Source: CAD feature listing. Evaluate the final solid. Frame: model axes, mm. A direction names the side the tool comes from. Coordinates: 2 decimals unless noted, no trailing zeros. Loops run counter-clockwise (first coordinate to the right, second up) from the corner with the lowest first, then second, coordinate; pieces in that order, holes last.
```python
from build123d import *

# Parameters (mm, degrees)
ESQUISSE1_W        = 5
ESQUISSE1_H        = 5
ESQUISSE1_W_2      = 7.5
ESQUISSE1_R        = 1.5
ESQUISSE1_R_2      = 0.875
ESQUISSE1_R_3      = 3.5
BOSS_EXTRU_1_DEPTH = 5


with BuildPart() as part:
    # Esquisse1 → Boss.-Extru.1 (new body)
    # profile 1 of 4: a face of its own
    with BuildSketch(Plane.XY):
        with BuildLine():
            Line((-8, 5), (-8, -10))
            Line((-8, -10), (18, -10))
            Line((18, -10), (18, 0))
            Line((18, 0), (25, 0))
            Line((25, 0), (30, 19))
            Line((30, 19), (45, 19))
            Line((45, 19), (45, 34))
            Line((45, 34), (60, 34))
            ThreePointArc((60, 34), (67.778174593, 52.778174593), (49, 45))
            Line((49, 45), (49, 40))
            Line((49, 40), (20, 40))
            Line((20, 40), (20, 45))
            Line((20, 45), (10, 45))
            Line((10, 45), (10, 40))
            Line((10, 40), (5, 40))
            Line((5, 40), (5, 45))
            Line((5, 45), (-5, 45))
            Line((-5, 45), (-5, 40))
            Line((-5, 40), (-15, 40))
            Line((-15, 40), (-15, 21))
            Line((-15, 21), (-6, 21))
            Line((-6, 21), (-6, 24))
            Line((-6, 24), (9, 24))
            Line((9, 24), (9, 21))
            Line((9, 21), (17, 21))
            Line((17, 21), (17, 13))
            Line((17, 13), (13, 13))
            Line((13, 13), (13, 7))
            Line((13, 7), (9, 7))
            Line((9, 7), (9, 4))
            Line((9, 4), (0, 4))
            Line((0, 4), (0, 5))
            Line((0, 5), (-8, 5))
        make_face()
        with Locations((-2.5, -2.5)):
            Rectangle(ESQUISSE1_W, ESQUISSE1_H, mode=Mode.SUBTRACT)
        with Locations((9.25, -2.5)):
            Rectangle(ESQUISSE1_W_2, ESQUISSE1_H, mode=Mode.SUBTRACT)
        with Locations((35, 25)):
            Circle(ESQUISSE1_R, mode=Mode.SUBTRACT)
        with Locations((56.75, 37.35)):
            Circle(ESQUISSE1_R_2, mode=Mode.SUBTRACT)
        with Locations((60, 45)):
            Circle(ESQUISSE1_R_3, mode=Mode.SUBTRACT)
        with Locations((67.65, 41.75)):
            Circle(ESQUISSE1_R_2, mode=Mode.SUBTRACT)
        with Locations((52.35, 48.25)):
            Circle(ESQUISSE1_R_2, mode=Mode.SUBTRACT)
        with Locations((63.25, 52.65)):
            Circle(ESQUISSE1_R_2, mode=Mode.SUBTRACT)
    # profile 2 of 4: a face of its own
    with BuildSketch(Plane.XY):
        with BuildLine():
            Line((-8, 5), (-8, -10))
            Line((-8, -10), (18, -10))
            Line((18, -10), (18, 0))
            Line((18, 0), (25, 0))
            Line((25, 0), (30, 19))
            Line((30, 19), (45, 19))
            Line((45, 19), (45, 34))
            Line((45, 34), (60, 34))
            ThreePointArc((60, 34), (67.778174593, 52.778174593), (49, 45))
            Line((49, 45), (49, 40))
            Line((49, 40), (20, 40))
            Line((20, 40), (20, 45))
            Line((20, 45), (10, 45))
            Line((10, 45), (10, 40))
            Line((10, 40), (5, 40))
            Line((5, 40), (5, 45))
            Line((5, 45), (-5, 45))
            Line((-5, 45), (-5, 40))
            Line((-5, 40), (-15, 40))
            Line((-15, 40), (-15, 21))
            Line((-15, 21), (-6, 21))
            Line((-6, 21), (-6, 24))
            Line((-6, 24), (9, 24))
            Line((9, 24), (9, 21))
            Line((9, 21), (17, 21))
            Line((17, 21), (17, 13))
            Line((17, 13), (13, 13))
            Line((13, 13), (13, 7))
            Line((13, 7), (9, 7))
            Line((9, 7), (9, 4))
            Line((9, 4), (0, 4))
            Line((0, 4), (0, 5))
            Line((0, 5), (-8, 5))
        make_face()
        with Locations((-2.5, -2.5)):
            Rectangle(ESQUISSE1_W, ESQUISSE1_H, mode=Mode.SUBTRACT)
        with Locations((9.25, -2.5)):
            Rectangle(ESQUISSE1_W_2, ESQUISSE1_H, mode=Mode.SUBTRACT)
        with Locations((35, 25)):
            Circle(ESQUISSE1_R, mode=Mode.SUBTRACT)
        with Locations((56.75, 37.35)):
            Circle(ESQUISSE1_R_2, mode=Mode.SUBTRACT)
        with Locations((60, 45)):
            Circle(ESQUISSE1_R_3, mode=Mode.SUBTRACT)
        with Locations((67.65, 41.75)):
            Circle(ESQUISSE1_R_2, mode=Mode.SUBTRACT)
        with Locations((52.35, 48.25)):
            Circle(ESQUISSE1_R_2, mode=Mode.SUBTRACT)
        with Locations((63.25, 52.65)):
            Circle(ESQUISSE1_R_2, mode=Mode.SUBTRACT)
    # profile 3 of 4: a face of its own
    with BuildSketch(Plane.XY):
        with BuildLine():
            Line((-8, 5), (-8, -10))
            Line((-8, -10), (18, -10))
            Line((18, -10), (18, 0))
            Line((18, 0), (25, 0))
            Line((25, 0), (30, 19))
            Line((30, 19), (45, 19))
            Line((45, 19), (45, 34))
            Line((45, 34), (60, 34))
            ThreePointArc((60, 34), (67.778174593, 52.778174593), (49, 45))
            Line((49, 45), (49, 40))
            Line((49, 40), (20, 40))
            Line((20, 40), (20, 45))
            Line((20, 45), (10, 45))
            Line((10, 45), (10, 40))
            Line((10, 40), (5, 40))
            Line((5, 40), (5, 45))
            Line((5, 45), (-5, 45))
            Line((-5, 45), (-5, 40))
            Line((-5, 40), (-15, 40))
            Line((-15, 40), (-15, 21))
            Line((-15, 21), (-6, 21))
            Line((-6, 21), (-6, 24))
            Line((-6, 24), (9, 24))
            Line((9, 24), (9, 21))
            Line((9, 21), (17, 21))
            Line((17, 21), (17, 13))
            Line((17, 13), (13, 13))
            Line((13, 13), (13, 7))
            Line((13, 7), (9, 7))
            Line((9, 7), (9, 4))
            Line((9, 4), (0, 4))
            Line((0, 4), (0, 5))
            Line((0, 5), (-8, 5))
        make_face()
        with Locations((-2.5, -2.5)):
            Rectangle(ESQUISSE1_W, ESQUISSE1_H, mode=Mode.SUBTRACT)
        with Locations((9.25, -2.5)):
            Rectangle(ESQUISSE1_W_2, ESQUISSE1_H, mode=Mode.SUBTRACT)
        with Locations((35, 25)):
            Circle(ESQUISSE1_R, mode=Mode.SUBTRACT)
        with Locations((56.75, 37.35)):
            Circle(ESQUISSE1_R_2, mode=Mode.SUBTRACT)
        with Locations((60, 45)):
            Circle(ESQUISSE1_R_3, mode=Mode.SUBTRACT)
        with Locations((67.65, 41.75)):
            Circle(ESQUISSE1_R_2, mode=Mode.SUBTRACT)
        with Locations((52.35, 48.25)):
            Circle(ESQUISSE1_R_2, mode=Mode.SUBTRACT)
        with Locations((63.25, 52.65)):
            Circle(ESQUISSE1_R_2, mode=Mode.SUBTRACT)
    # profile 4 of 4: a face of its own
    with BuildSketch(Plane.XY):
        with BuildLine():
            Line((-8, 5), (-8, -10))
            Line((-8, -10), (18, -10))
            Line((18, -10), (18, 0))
            Line((18, 0), (25, 0))
            Line((25, 0), (30, 19))
            Line((30, 19), (45, 19))
            Line((45, 19), (45, 34))
            Line((45, 34), (60, 34))
            ThreePointArc((60, 34), (67.778174593, 52.778174593), (49, 45))
            Line((49, 45), (49, 40))
            Line((49, 40), (20, 40))
            Line((20, 40), (20, 45))
            Line((20, 45), (10, 45))
            Line((10, 45), (10, 40))
            Line((10, 40), (5, 40))
            Line((5, 40), (5, 45))
            Line((5, 45), (-5, 45))
            Line((-5, 45), (-5, 40))
            Line((-5, 40), (-15, 40))
            Line((-15, 40), (-15, 21))
            Line((-15, 21), (-6, 21))
            Line((-6, 21), (-6, 24))
            Line((-6, 24), (9, 24))
            Line((9, 24), (9, 21))
            Line((9, 21), (17, 21))
            Line((17, 21), (17, 13))
            Line((17, 13), (13, 13))
            Line((13, 13), (13, 7))
            Line((13, 7), (9, 7))
            Line((9, 7), (9, 4))
            Line((9, 4), (0, 4))
            Line((0, 4), (0, 5))
            Line((0, 5), (-8, 5))
        make_face()
        with Locations((-2.5, -2.5)):
            Rectangle(ESQUISSE1_W, ESQUISSE1_H, mode=Mode.SUBTRACT)
        with Locations((9.25, -2.5)):
            Rectangle(ESQUISSE1_W_2, ESQUISSE1_H, mode=Mode.SUBTRACT)
        with Locations((35, 25)):
            Circle(ESQUISSE1_R, mode=Mode.SUBTRACT)
        with Locations((56.75, 37.35)):
            Circle(ESQUISSE1_R_2, mode=Mode.SUBTRACT)
        with Locations((60, 45)):
            Circle(ESQUISSE1_R_3, mode=Mode.SUBTRACT)
        with Locations((67.65, 41.75)):
            Circle(ESQUISSE1_R_2, mode=Mode.SUBTRACT)
        with Locations((52.35, 48.25)):
            Circle(ESQUISSE1_R_2, mode=Mode.SUBTRACT)
        with Locations((63.25, 52.65)):
            Circle(ESQUISSE1_R_2, mode=Mode.SUBTRACT)
    extrude(amount=BOSS_EXTRU_1_DEPTH)


solid = part.part
```
Q1. Section query D-D on y = 12. Return the cut outline in (x, z).
Q2. Draft query along Y for faces 1 (the flat face through (-10, 40, 2)), 2 (the flat face through (0, -3, 2)), 3 (the flat face through (49, 43, 2)). Return one class per face: released by +Y, released by -Y, zero draft, split by the parting line, or undercut.
Q3. Section query C-C on z = 2.15. Count the separate pieces of the cut face and the enclosed holes in it, then the cut area to 3 significant figures.
Q4. Section query B-B on y = 37.35. Return the cut outline in (x, z) (3 decimals).
Q5. First-contact query: pin 1 Ø2 at (y, z) = (12.5, 2.5) entering from -X; pin 2 Ø1.5 at (y, z) = (-3, 2) entering from -X; pin 3 Ø1.5 at (y, z) = (22.5, 3) entering from +X; pin 4 Ø10 at (x, y) = (33, 3) entering from +Z. Flat tips, straight axial feed; report the tip coordinate or a pass-through.
Q6. Material intervals for line 1 along Y through (x, z) = (35, 3.95); line 2 along Y through (x, z) = (3, 1.1); line 3 along X through (y, z) = (27, 1.75), sorted ascending.
Q7. Reachability of faces 4 (the flat face through (13, -3, 2)), 5 (the flat face through (35, 40, 2)), 6 (the flat face through (45, 26, 2)) from +Z, -Z, +X, -X, +Y, -Y: full face, straight path, thin tool, end or side. Return the list, or none.
Q8. Section query A-A on x = 35. Return the cut outline in (y, z).
Resolved:
1. outline: (13, 0) - (28.16, 0) - (28.16, 5) - (13, 5) - close
2. face 1: released by +Y
2. face 2: undercut
2. face 3: zero draft
3. separate pieces: 1
3. enclosed holes: 8
3. area: 2,180 mm2
4. outline: (-15, 0) - (55.875, 0) - (55.875, 5) - (-15, 5) - close; (57.625, 0) - (67.904, 0) - (67.904, 5) - (57.625, 5) - close
5. pin 1: stops at x = 13
5. pin 2: stops at x = -8
5. pin 3: stops at x = 45
5. pin 4: passes through
6. line 1: y = 19 to 23.5, 26.5 to 40
6. line 2: y = -10 to 4, 24 to 45
6. line 3: x = -15 to 45
7. face 4: +Z, -Z
7. face 5: +Z, -Z, +Y
7. face 6: +Z, -Z, +X, -Y
8. outline: (19, 0) - (23.5, 0) - (23.5, 5) - (19, 5) - close; (26.5, 0) - (40, 0) - (40, 5) - (26.5, 5) - close
